Work out the finished part from the listing and answer in its coordinate system (mm). A direction names the side the tool comes from. Coordinates: 2 decimals unless noted, no trailing zeros. Order: outer loops, then holes, each group sorted by start corner. A loop starts at its lowest first (then second) coordinate and runs counter-clockwise, first axis right, second up. Notation, with made-up numbers: M 78.5,-23 L 84.5,-23 A22 ccw 84.5,13 Z; hole C 83.25,50.5 d4. An arc over 180 degrees is marked long. Answer in a Markdown table with one row per item. Add a question column.
Item 1: Flat-ended cylindrical pins translate along their axes: pin 1 Ø3 at (y, z) = (8.5, 6.5) entering from -X; pin 2 Ø8 at (x, z) = (53, 4.5) entering from +Y; pin 3 Ø14 at (x, z) = (-31, 3) entering from +Y. Find the tip coordinate at first contact, or state that the pin passes through.
Item 2: The part is cut by section C-C (z = -4). Write down the section's boundary in (x, y).
Item 3: The part is cut by section A-A (y = 4). Write down the section's boundary in (x, z), then the cut area to 3 significant figures.
Item 4: Which of the six approach directions +Z, -Z, +X, -X, +Y, -Y give full straight-line access (tool end or side, diameter ignored) to faces 1 (the face through (73.57, 3.2, -16)), 2 (the face through (55.5, 6, 0))?
Item 5: The mould has two halves that part along X. Classify faces 3 (the face through (-1, 3, 17.5)), 4 (the face through (-38, 2, 0)), 5 (the face through (-74, 8.95, -0.18)): released by +X, released by -X, zero draft, split by the parting line, or undercut.
Item 6: Consider line 1 (X direction, y = 3, z = -1); line 2 (Z direction, x = 28.5, y = 4); line 3 (X direction, y = 8, z = 5). Determine where each line is inside the solid, lowest interval first. Write a range as from..to.
from build123d import *

# Parameters (mm, degrees)
SKETCH1_W           = 150
SKETCH1_H           = 35
SKETCH1_W_2         = 28
SKETCH1_H_2         = 28
SKETCH1_W_3         = 36
BOSS_EXTRUDE1_DEPTH = 10
SKETCH2_W           = 28
SKETCH2_H           = 28
SKETCH2_W_2         = 36
BOSS_EXTRUDE2_DEPTH = 2
FILLET3_R           = 3.5
FILLET4_R           = 5


# Some blends are built 0.0001 mm under size
with BuildPart() as part:
    # Sketch1 → Boss-Extrude1 (new body)
    with BuildSketch(Plane(origin=(0, 0, 0), x_dir=(1, 0, 0), z_dir=(0, 1, 0))):
        Rectangle(SKETCH1_W, SKETCH1_H)
        Rectangle(SKETCH1_W_2, SKETCH1_H_2, mode=Mode.SUBTRACT)
        with Locations((-37.5, 0)):
            Rectangle(SKETCH1_W_2, SKETCH1_H_2, mode=Mode.SUBTRACT)
        with Locations((37.5, 0)):
            Rectangle(SKETCH1_W_3, SKETCH1_H_2, mode=Mode.SUBTRACT)
    extrude(amount=BOSS_EXTRUDE1_DEPTH)

    # Sketch2 → Boss-Extrude2 (add)
    with BuildSketch(Plane.XZ):
        with Locations((-37.5, 0)):
            Rectangle(SKETCH2_W, SKETCH2_H)
        Rectangle(SKETCH2_W, SKETCH2_H)
        with Locations((37.5, 0)):
            Rectangle(SKETCH2_W_2, SKETCH2_H)
    extrude(amount=-BOSS_EXTRUDE2_DEPTH)

    # Fillet3
    fillet3_edges = [part.edges().sort_by_distance(p)[0] for p in [
        (-75, 10, 0),
        (0, 10, 17.5),
        (75, 10, 0),
        (0, 10, -17.5),
    ]]
    fillet(fillet3_edges, radius=FILLET3_R - 0.0001)  # a hair under: the kernel refuses the full size

    # Fillet4
    # the kernel refuses this fillet: 5 mm, written as the material it takes off along each edge
    with BuildSketch(Plane(origin=(70, 10, -12.5), x_dir=(1, 0, 0), z_dir=(0, 0, 1))) as fillet4_piece_1:
        with BuildLine():
            CenterArc((1.5001, -3.4999), 3.4999, 0, 90)
            Line((5, -3.4999), (5, 0))
            Line((5, 0), (1.5001, 0))
        make_face()
    revolve(axis=Axis((70, 10, -12.5), (0, 1, 0)), revolution_arc=90, mode=Mode.SUBTRACT)
    with BuildSketch(Plane(origin=(70, 10, 12.5), x_dir=(0, 0, 1), z_dir=(-1, 0, 0))) as fillet4_piece_2:
        with BuildLine():
            CenterArc((1.5001, -3.4999), 3.4999, 0, 90)
            Line((5, -3.4999), (5, 0))
            Line((5, 0), (1.5001, 0))
        make_face()
    revolve(axis=Axis((70, 10, 12.5), (0, 1, 0)), revolution_arc=90, mode=Mode.SUBTRACT)
    with BuildSketch(Plane(origin=(-70, 10, -12.5), x_dir=(0, 0, -1), z_dir=(1, 0, 0))) as fillet4_piece_3:
        with BuildLine():
            CenterArc((1.5001, -3.4999), 3.4999, 0, 90)
            Line((5, -3.4999), (5, 0))
            Line((5, 0), (1.5001, 0))
        make_face()
    revolve(axis=Axis((-70, 10, -12.5), (0, 1, 0)), revolution_arc=90, mode=Mode.SUBTRACT)
    with BuildSketch(Plane(origin=(-70, 10, 12.5), x_dir=(-1, 0, 0), z_dir=(0, 0, -1))) as fillet4_piece_4:
        with BuildLine():
            CenterArc((1.5001, -3.4999), 3.4999, 0, 90)
            Line((5, -3.4999), (5, 0))
            Line((5, 0), (1.5001, 0))
        make_face()
    revolve(axis=Axis((-70, 10, 12.5), (0, 1, 0)), revolution_arc=90, mode=Mode.SUBTRACT)
    with BuildSketch(Plane(origin=(-75, -12.5, 17.5), x_dir=(1, 0, 0), z_dir=(0, 1, 0)), Plane(origin=(-75, -12.5, -17.5), x_dir=(0, 0, 1), z_dir=(0, 1, 0))) as fillet4_piece_5:
        with BuildLine():
            CenterArc((FILLET4_R, FILLET4_R), FILLET4_R, 180, 90)
            Line((0, FILLET4_R), (0, 0))
            Line((0, 0), (FILLET4_R, 0))
        make_face()
    extrude(amount=22.5, mode=Mode.SUBTRACT)
    with BuildSketch(Plane(origin=(75, -12.5, -17.5), x_dir=(0, 0, 1), z_dir=(0, 1, 0)), Plane(origin=(75, -12.5, 17.5), x_dir=(-1, 0, 0), z_dir=(0, 1, 0))) as fillet4_piece_6:
        with BuildLine():
            CenterArc((FILLET4_R, -FILLET4_R), FILLET4_R, 90, 90)
            Line((0, -FILLET4_R), (0, 0))
            Line((0, 0), (FILLET4_R, 0))
        make_face()
    extrude(amount=22.5, mode=Mode.SUBTRACT)


solid = part.part
Reply:
| question | item | result |
|---|---|---|
| 1 | pin 1 | stops at x = -74.96 |
| 1 | pin 2 | stops at y = 10 |
| 1 | pin 3 | stops at y = 2 |
| 2 | outline | M -75,0 L 75,0 L 75,6.5 A3.5 ccw 71.5,10 L 55.5,10 L 55.5,2 L 19.5,2 L 19.5,10 L 14,10 L 14,2 L -14,2 L -14,10 L -23.5,10 L -23.5,2 L -51.5,2 L -51.5,10 L -71.5,10 A3.5 ccw -75,6.5 Z |
| 3 | outline | M -75,-12.5 A5 ccw -70,-17.5 L 70,-17.5 A5 ccw 75,-12.5 L 75,12.5 A5 ccw 70,17.5 L -70,17.5 A5 ccw -75,12.5 Z; hole M -51.5,-14 L -23.5,-14 L -23.5,14 L -51.5,14 Z; hole M -14,-14 L 14,-14 L 14,14 L -14,14 Z; hole M 19.5,-14 L 55.5,-14 L 55.5,14 L 19.5,14 Z |
| 3 | area | 2,650 mm2 |
| 4 | face 1 | -Z, +X, +Y, -Y |
| 4 | face 2 | +Y |
| 5 | face 3 | zero draft |
| 5 | face 4 | undercut |
| 5 | face 5 | released by -X |
| 6 | line 1 | x = -75..-51.5, -23.5..-14, 14..19.5, 55.5..75 |
| 6 | line 2 | z = -17.5..-14, 14..17.5 |
| 6 | line 3 | x = -74.66..-51.5, -23.5..-14, 14..19.5, 55.5..74.66 |
